For this review, take the finished solid that the model builds, in its own axes (mm). A direction names the side the tool comes from. Coordinates: 2 decimals unless noted, no trailing zeros.
1. Clearance check with a flat-ended pin moving along its axis: P1, Ø1, axis at x = 0.5, y = -3.5, coming from the +Z side. State where the tip first meets the part, or that it passes through.
2. Mouldability with a two-part tool opening along Y and no side actions: class faces 3 (the face through (0, -10, 1143)), 4 (the face through (0, 2, 1290)), 5 (the face through (-1, -8.5, 1143)), 6 (the face through (6, 10, 1143)) as pulls with the +Y half, pulls with the -Y half, needs draft (parallel to the pull), parting line crosses it, or undercut.
3. To check wall thickness, follow probe 1 along X at (y, z) = (2.5, 1061); probe 2 along Y at (x, z) = (-7, 1091); probe 3 along Y at (x, z) = (2.5, 1163.5). State the ranges of each line that lie inside material, in increasing order.
4. Take a section at A-A, the plane z = 1155.5. Count the separate pieces of the cut face and the enclosed holes in it, then the cut area to 3 significant figures.
5. Machinability: for faces 1 (the face through (8.5, 1, 1143)), 2 (the face through (10, 0, 1143)), which of the approach directions +Z, -Z, +X, -X, +Y, -Y give a long, thin tool a straight path to every point of the face, cutting with its end or side? Answer none if there is none.
Autodesk Inventor part; units mm, degrees
ref_plane "作業平面1" through (-9.5, -10, 1000) normal (0, 0, 1) x (1, 0, 0)
ref_plane "YZ Plane" through (0, 0, 0) normal (1, 0, 0) x (0, 1, 0)
ref_plane "XZ Plane" through (0, 0, 0) normal (0, 1, 0) x (-1, 0, 0)
ref_plane "作業平面1" through (-9.5, -10, 1000) normal (0, 0, 1) x (1, 0, 0)
sketch "スケッチ1" plane through (-9.5, -10, 1000) normal (0, 0, 1) x (1, 0, 0)
  line L0 (7.35, 18.5) -> (7.35, 20)
  line L1 (7.35, 20) -> (0, 20)
  arc A0 (0, 20) -> (-0.5, 19.5) centre (0, 19.5) ccw
  line L2 (-0.5, 19.5) -> (-0.5, 12.15)
  line L3 (-0.5, 12.15) -> (1, 12.15)
  line L4 (1, 12.15) -> (1, 14.15)
  line L5 (1, 14.15) -> (4.7, 14.15)
  line L6 (4.7, 14.15) -> (4.7, 12.15)
  line L7 (4.7, 12.15) -> (6.5, 12.15)
  line L8 (6.5, 12.15) -> (6.5, 7.85)
  line L9 (6.5, 7.85) -> (4.7, 7.85)
  line L10 (4.7, 7.85) -> (4.7, 5.85)
  line L11 (4.7, 5.85) -> (1, 5.85)
  line L12 (1, 5.85) -> (1, 7.85)
  line L13 (1, 7.85) -> (-0.5, 7.85)
  line L14 (-0.5, 7.85) -> (-0.5, 0.5)
  arc A1 (-0.5, 0.5) -> (0, 0) centre (0, 0.5) ccw
  line L15 (0, 0) -> (19, 0)
  arc A2 (19, 0) -> (19.5, 0.5) centre (19, 0.5) ccw
  line L16 (19.5, 0.5) -> (19.5, 19.5)
  arc A3 (19.5, 19.5) -> (19, 20) centre (19, 19.5) ccw
  line L17 (19, 20) -> (11.65, 20)
  line L18 (11.65, 20) -> (11.65, 18.5)
  line L19 (11.65, 18.5) -> (13.65, 18.5)
  line L20 (13.65, 18.5) -> (13.65, 14.8)
  line L21 (13.65, 14.8) -> (11.65, 14.8)
  line L22 (11.65, 14.8) -> (11.65, 13)
  line L23 (11.65, 13) -> (7.35, 13)
  line L24 (7.35, 13) -> (7.35, 14.8)
  line L25 (7.35, 14.8) -> (5.35, 14.8)
  line L26 (5.35, 14.8) -> (5.35, 18.5)
  line L27 (5.35, 18.5) -> (7.35, 18.5)
  arc A4 (17.7174, 15.4132) -> (17.6402, 15.0252) centre (17.9, 15.1752) ccw
  line L28 (17.6402, 15.0252) -> (17.9598, 14.4715)
  arc A5 (18, 14.3215) -> (17.9598, 14.4715) centre (17.7, 14.3215) ccw
  line L29 (18, 14.3215) -> (18, 6.7162)
  arc A6 (17.7225, 6.4162) -> (18, 6.7162) centre (17.7, 6.7153) ccw
  line L30 (17.7225, 6.4162) -> (17.0355, 6.4162)
  arc A7 (17.0355, 6.4162) -> (16.8233, 6.3283) centre (17.0355, 6.1162) ccw
  line L31 (16.8233, 6.3283) -> (15.9875, 5.4924)
  arc A8 (15.9875, 5.4924) -> (16.2388, 4.9829) centre (16.1996, 5.2803) ccw
  arc A9 (14.5171, 3.2612) -> (16.2388, 4.9829) centre (16.5, 3) ccw
  arc A10 (14.5171, 3.2612) -> (14.2973, 3.5902) centre (14.2197, 3.3004) ccw
  line L32 (14.2973, 3.5902) -> (14.2135, 3.6127)
  arc A11 (14.2135, 3.6127) -> (13.9237, 3.535) centre (14.1359, 3.3229) ccw
  line L33 (13.9237, 3.535) -> (13.0879, 2.6991)
  arc A12 (13.0879, 2.6991) -> (13, 2.487) centre (13.3, 2.487) ccw
  line L34 (13, 2.487) -> (13, 1.8)
  arc A13 (12.7, 1.5) -> (13, 1.8) centre (12.7, 1.8) ccw
  line L35 (12.7, 1.5) -> (5.1785, 1.5)
  arc A14 (5.0285, 1.5402) -> (5.1785, 1.5) centre (5.1785, 1.8) ccw
  line L36 (5.0285, 1.5402) -> (4.4748, 1.8598)
  arc A15 (4.4748, 1.8598) -> (4.0868, 1.7826) centre (4.3248, 1.6) ccw
  arc A16 (4.0868, 4.2174) -> (4.0868, 1.7826) centre (2.5, 3) ccw
  arc A17 (4.0868, 4.2174) -> (4.4748, 4.1402) centre (4.3248, 4.4) ccw
  line L37 (4.4748, 4.1402) -> (6.2409, 5.1598)
  arc A18 (6.3909, 5.2) -> (6.2409, 5.1598) centre (6.3909, 4.9) ccw
  line L38 (6.3909, 5.2) -> (7.05, 5.2)
  arc A19 (7.05, 5.2) -> (7.35, 5.5) centre (7.05, 5.5) ccw
  line L39 (7.35, 5.5) -> (7.35, 6.4)
  arc A20 (7.95, 7) -> (7.35, 6.4) centre (7.95, 6.4) ccw
  line L40 (7.95, 7) -> (9.2042, 7)
  arc A21 (9.2042, 7) -> (9.4163, 7.0879) centre (9.2042, 7.3) ccw
  line L41 (9.4163, 7.0879) -> (9.9752, 7.6468)
  arc A22 (9.9752, 7.6468) -> (10.0529, 7.9366) centre (9.7631, 7.8589) ccw
  line L42 (10.0529, 7.9366) -> (9.9987, 8.1389)
  arc A23 (9.9987, 8.1389) -> (9.6768, 8.3595) centre (9.7089, 8.0612) ccw
  arc A24 (11.1405, 9.8232) -> (9.6768, 8.3595) centre (9.5, 10) ccw
  arc A25 (11.1405, 9.8232) -> (11.3611, 9.5013) centre (11.4388, 9.7911) ccw
  line L43 (11.3611, 9.5013) -> (11.5634, 9.4471)
  arc A26 (11.5634, 9.4471) -> (11.8532, 9.5248) centre (11.6411, 9.7369) ccw
  line L44 (11.8532, 9.5248) -> (12.4121, 10.0837)
  arc A27 (12.4121, 10.0837) -> (12.5, 10.2958) centre (12.2, 10.2958) ccw
  line L45 (12.5, 10.2958) -> (12.5, 11.55)
  arc A28 (13.1, 12.15) -> (12.5, 11.55) centre (13.1, 11.55) ccw
  line L46 (13.1, 12.15) -> (14, 12.15)
  arc A29 (14, 12.15) -> (14.2652, 12.4701) centre (13.966, 12.4481) ccw
  line L47 (14.2652, 12.4701) -> (14.2652, 13.0488)
  arc A30 (14.3054, 13.1988) -> (14.2652, 13.0488) centre (14.5652, 13.0488) ccw
  line L48 (14.3054, 13.1988) -> (15.3598, 15.0252)
  arc A31 (15.3598, 15.0252) -> (15.2826, 15.4132) centre (15.1, 15.1752) ccw
  arc A32 (17.7174, 15.4132) -> (15.2826, 15.4132) centre (16.5, 17) ccw
  circle A33 centre (2.5, 17) radius 2
  point P0 (9.5, 10)
extrude "押し出し1" add sketch "スケッチ1" along normal blind 290
properties part number "AFST-2020-4-1000"
Results list:
1. P1: passes through
2. face 3: pulls with the -Y half
2. face 4: needs draft
2. face 5: undercut
2. face 6: pulls with the +Y half
3. probe 1: x = -10 to -8.5, -4.8 to 4.77, 8.5 to 10
3. probe 2: y = -10 to -9, -5 to -4.15, 4.15 to 5, 9 to 10
3. probe 3: y = -10 to -8.5, -0.33 to 4.8, 8.5 to 10
4. separate pieces: 1
4. enclosed holes: 2
4. area: 155 mm2
5. face 1: +Z, -Z
5. face 2: +Z, -Z, +X, +Y, -Y
